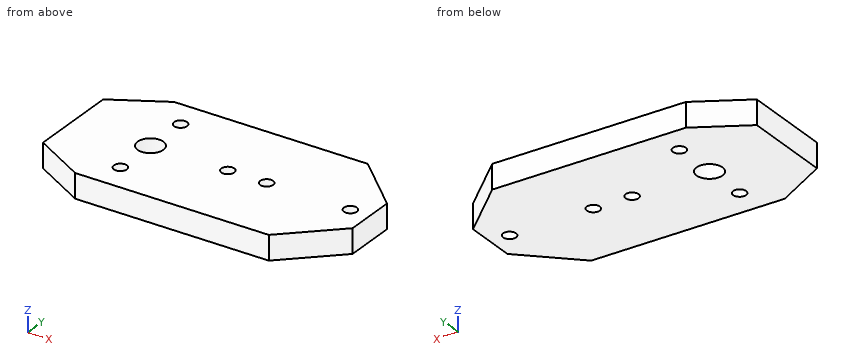
from build123d import *

# Parameters (mm, degrees)
SKETCH1_R           = 1.6
SKETCH1_R_2         = 3.175
BOSS_EXTRUDE1_DEPTH = 6


with BuildPart() as part:
    # Sketch1 → Boss-Extrude1 (new body)
    with BuildSketch(Plane.XY):
        Polygon((-19.05, -11.1), (-6.35, -18.25), (41.3, -18.25), (53.975, -6.35), (53.975, 6.35), (41.3, 18.25), (-6.35, 18.25), (-19.05, 11.1), align=None)
        with Locations((19.05, 0)):
            Circle(SKETCH1_R, mode=Mode.SUBTRACT)
        with Locations((28.6, 0)):
            Circle(SKETCH1_R, mode=Mode.SUBTRACT)
        with Locations((49.2, 0)):
            Circle(SKETCH1_R, mode=Mode.SUBTRACT)
        Circle(SKETCH1_R_2, mode=Mode.SUBTRACT)
        with Locations((0, 11.1)):
            Circle(SKETCH1_R, mode=Mode.SUBTRACT)
        with Locations((0, -11.1)):
            Circle(SKETCH1_R, mode=Mode.SUBTRACT)
    extrude(amount=BOSS_EXTRUDE1_DEPTH)


solid = part.part
The model under review builds one solid part; all positions refer to its coordinate system, in mm. Give positions to 0.01 mm unless a question says otherwise; leave off trailing zeros. Write each loop counter-clockwise with the first axis right and the second up, starting at its lowest first coordinate (ties: lowest second). Pieces come first, ordered by that corner, then holes. Notation, with made-up numbers: M 43.5,75 L 70.5,75 A19 ccw 70.5,83 Z; hole C 12.5,17.25 d1. An arc over 180 degrees is marked long. One line per question, with ' | ' between items. Start each with the question number.
Item 1: Wall thickness on line 1 (Y direction, x = 0, z = 3.7) (3 decimals); line 2 (Y direction, x = 19.05, z = 2.15); line 3 (X direction, y = -0.5, z = 1.9) (3 decimals): over which ranges is each line inside the solid? List them lowest first. Write a range as from..to.
Item 2: We need section A-A on y = 0. Write out the cut boundary in (x, z) (3 decimals).
Item 3: For pin 1 (1.9 mm diameter, centred on x = 49.2, y = 0, fed in from -Z); pin 2 (3 mm diameter, centred on y = -13.5, z = 1.5, fed in from -X), all flat-tipped, find the tip position at first contact; note any pin that passes through.
Item 4: We need section D-D on x = 49.2. Write out the cut boundary in (y, z).
Item 5: We need section C-C on z = 2.2. Write out the cut boundary in (x, y) (3 decimals), plus the area to 3 significant figures.
Item 6: We need section B-B on x = 19.05. Write out the cut boundary in (y, z).
Results found:
1) line 1: y = -18.25..-12.7, -9.5..-3.175, 3.175..9.5, 12.7..18.25 | line 2: y = -18.25..-1.6, 1.6..18.25 | line 3: x = -19.05..-3.135, 3.135..17.53, 20.57..27.08, 30.12..47.68, 50.72..53.975
2) outline: M -19.05,0 L -3.175,0 L -3.175,6 L -19.05,6 Z; M 3.175,0 L 17.45,0 L 17.45,6 L 3.175,6 Z; M 20.65,0 L 27,0 L 27,6 L 20.65,6 Z; M 30.2,0 L 47.6,0 L 47.6,6 L 30.2,6 Z; M 50.8,0 L 53.975,0 L 53.975,6 L 50.8,6 Z
3) pin 1: passes through | pin 2: stops at x = -17.45
4) outline: M -10.83,0 L -1.6,0 L -1.6,6 L -10.83,6 Z; M 1.6,0 L 10.83,0 L 10.83,6 L 1.6,6 Z
5) outline: M -19.05,-11.1 L -6.35,-18.25 L 41.3,-18.25 L 53.975,-6.35 L 53.975,6.35 L 41.3,18.25 L -6.35,18.25 L -19.05,11.1 Z; hole C 0,0 d6.35; hole C 0,-11.1 d3.2; hole C 0,11.1 d3.2; hole C 19.05,0 d3.2; hole C 28.6,0 d3.2; hole C 49.2,0 d3.2 | area: 2,350 mm2
6) outline: M -18.25,0 L -1.6,0 L -1.6,6 L -18.25,6 Z; M 1.6,0 L 18.25,0 L 18.25,6 L 1.6,6 Z
